Geometry: final body of the model. Coordinates: model frame, mm. A direction names the side the tool comes from. Coordinates: 2 decimals unless noted, no trailing zeros. Write each loop counter-clockwise with the first axis right and the second up, starting at its lowest first coordinate (ties: lowest second). Pieces come first, ordered by that corner, then holes.
from build123d import *

# Parameters (mm, degrees)
F1_DEPTH = 5
F2_R     = 1
F4_START = 5
F4_DEPTH = 15
F5_R     = 1


with BuildPart() as f1:
    # F0 (on Top) → F1 (new body)
    with BuildSketch(Plane.XY):
        with BuildLine():
            Line((2.3027157879, 2), (4.9135552302, 2))
            ThreePointArc((4.9135552302, 2), (-5.305, 0), (4.9135552302, -2))
            Line((4.9135552302, -2), (2.3027157879, -2))
            ThreePointArc((2.3027157879, -2), (-3.05, 0), (2.3027157879, 2))
        make_face()
    extrude(amount=F1_DEPTH)

    # F2
    f2_edges = [f1.edges().sort_by_distance(p)[0] for p in [
        (4.913555, 2, 2.5),
        (2.302716, 2, 2.5),
        (2.302716, -2, 2.5),
        (4.913555, -2, 2.5),
    ]]
    fillet(f2_edges, radius=F2_R)

    # F3 (on Top) → F4 (join)
    with BuildSketch(Plane.XY.offset(F4_START)):
        with BuildLine():
            Line((2.655654345, 1.5), (5.0885189397, 1.5))
            ThreePointArc((5.0885189397, 1.5), (-5.305, 0), (5.0885189397, -1.5))
            Line((5.0885189397, -1.5), (2.655654345, -1.5))
            ThreePointArc((2.655654345, -1.5), (-3.05, 0), (2.655654345, 1.5))
        make_face()
    extrude(amount=F4_DEPTH)

    # F5
    f5_edges = [f1.edges().sort_by_distance(p)[0] for p in [
        (5.088519, -1.5, 12.5),
        (5.088519, 1.5, 12.5),
        (2.655654, -1.5, 12.5),
        (2.655654, 1.5, 12.5),
    ]]
    fillet(f5_edges, radius=F5_R)


solid = f1.part
Item 1: Material intervals for probe 1 along Y at (x, z) = (0, 2.2) (3 decimals); probe 2 along Y at (x, z) = (3.25, 9); probe 3 along X at (y, z) = (2.25, 5.75), sorted ascending.
Derived:
probe 1: y = -5.305 to -3.05, 3.05 to 5.305
probe 2: y = -4.19 to -1.5, 1.5 to 4.19
probe 3: x = -4.8 to -2.06, 2.06 to 4.47
Item 2: Pull-direction query (Y, two-part tool) for faces 1 (the flat face through (-3, -2, 0)), 2 (the cylindrical face through (4.401, -2.056, 12.605)); classes: released by +Y, released by -Y, zero draft, split by the parting line, or undercut.
Derived:
face 1: zero draft
face 2: undercut
Item 3: Section C-C, the plane y = -2.5. Output: boundary loops of the cut face in (x, z), plus the area to 3 significant figures.
Derived:
outline: (-4.68, 0) - (-1.75, 0) - (-1.75, 20) - (-4.68, 20) - close; (1.75, 0) - (3.95, 0) - (3.95, 5) - (4.5, 5) - (4.5, 20) - (1.75, 20) - close
area: 111 mm2
Item 4: Section A-A, the plane x = 0. Output: boundary loops of the cut face in (y, z) (3 decimals).
Derived:
outline: (-5.305, 0) - (-3.05, 0) - (-3.05, 20) - (-5.305, 20) - close; (3.05, 0) - (5.305, 0) - (5.305, 20) - (3.05, 20) - close
Item 5: Section B-B, the plane z = 5.75. Output: boundary loops of the cut face in (x, y) (3 decimals), plus the area to 3 significant figures.
Derived:
outline: (2.4, -1.883) arc R3.05 cw (long way) to (2.4, 1.883) arc R1 ccw to (3.186, 1.5) - (3.505, 1.5) arc R1 ccw to (4.319, 3.081) arc R5.305 ccw (long way) to (4.319, -3.081) arc R1 ccw to (3.505, -1.5) - (3.186, -1.5) arc R1 ccw to start
area: 50.9 mm2
Item 6: Set-up query: faces 3 (the cylindrical face through (4.002, 2.596, 2.535)), 4 (the cylindrical face through (4.387, 2.029, 12.605)). Return all of +Z, -Z, +X, -X, +Y, -Y with unobstructed straight access to the full face (end or side cutting, diameter ignored); none if empty.
Derived:
face 3: -Z, +X
face 4: +Z, -Z, +X
Item 7: Section D-D, the plane x = -2.5. Output: boundary loops of the cut face in (y, z).
Derived:
outline: (-4.68, 0) - (-1.75, 0) - (-1.75, 20) - (-4.68, 20) - close; (1.75, 0) - (4.68, 0) - (4.68, 20) - (1.75, 20) - close
Item 8: Pin query (flat end, axial travel): pin 1 (1 mm diameter, centred on x = 3.5, y = 4, fed in from -Z); pin 2 (4 mm diameter, centred on x = -3, z = 4.5, fed in from +Y). Return the tip coordinate at first contact, or that it passes through.
Derived:
pin 1: stops at z = 0
pin 2: stops at y = 5.21
